Autodesk Fusion 360 part; units mm, degrees
sketch "Sketch1" plane through (0, 0, 0) normal (0, 1, 0) x (1, 0, 0)
  line L0 (-10, 0) -> (17, 0)
  line L1 (17, 0) -> (17, -21.946)
  line L2 (17, -21.946) -> (-10, -21.946)
  line L3 (-10, -21.946) -> (-10, 0)
  dimension "d1" = 21.946
  dimension "d2" = 27
  dimension "d3" = 10
  dimension "d4" = 21.946
extrude "Extrude1" add sketch "Sketch1" along normal blind 5
sketch "Sketch2" plane through (0, 0, 0) normal (0, -1, 0) x (1, 0, 0)
  line L0 (17, 21.946) -> (-10, 21.946)
  line L1 (-10, 21.946) -> (-10, 0)
  line L2 (-10, 0) -> (17, 0)
  line L3 (17, 0) -> (17, 21.946)
  circle A0 centre (3.5, 21.946) radius 13.5
  circle A1 centre (3.5, 21.946) radius 12
  dimension "d7" = 27
  dimension "d8" = 24
extrude "Extrude2" add sketch "Sketch2" against normal blind 5 contours L0 A0 A1 picked at (13.449, 30.2624)
extrude "Extrude3" cut sketch "Sketch2" against normal blind 5 contours L0 A1 picked at (6.689, 16.5654)
equation "d1 = 21.616 mm + 0.33 mm"
equation "d4 = 21.616 mm + 0.33 mm"
Could you check a few things on this model? Use its own coordinates, in mm. Round coordinates to 2 decimals unless told otherwise and drop trailing zeros. Order: outer loops, then holes, each group sorted by start corner. A loop starts at its lowest first (then second) coordinate and runs counter-clockwise, first axis right, second up. Notation, with made-up numbers: M 67,-31.5 L 72,-31.5 A17 ccw 72,-15.5 Z; hole C 29,38.25 d3. An arc over 180 degrees is marked long. One line per item, written item: value.
(1) Imagine slicing it at A-A (x = 3.5). Write out the boundary of the cut face in (y, z), and give its area (3 significant figures).
Ans:
outline: M 0,0 L 5,0 L 5,9.95 L 0,9.95 Z; M 0,33.95 L 5,33.95 L 5,35.45 L 0,35.45 Z
area: 57.2 mm^2
(2) If we mould it in two halves opening along X, with no side actions, what happens to faces 1 (the cylindrical face through (1.938, 2.465, 33.844)), 2 (the flat face through (3.3, 0, 9.6)), 3 (the cylindrical face through (3.797, 2.465, 35.443)), 4 (the flat face through (17, 2, 11))? For each: released by +X, released by -X, zero draft, split by the parting line, or undercut.
Ans:
face 1: undercut
face 2: zero draft
face 3: split by the parting line
face 4: released by +X
(3) I need wall thicknesses on line 1 along Z through (x, y) = (3.5, 2.3); line 2 along Z through (x, y) = (2.75, 3.25); line 3 along X through (y, z) = (4.25, 28.5). Which ranges of each line are inside material? Lowest first, please. Write a range as from..to.
Ans:
line 1: z = 0..9.95, 33.95..35.45
line 2: z = 0..9.97, 33.92..35.43
line 3: x = -8.3..-6.55, 13.55..15.3
(4) Imagine slicing it at C-C (y = 0.65). Write out the boundary of the cut face in (x, z), and give its area (3 significant figures).
Ans:
outline: M -10,0 L 17,0 L 17,21.95 A13.5 ccw -10,21.95 Z; hole C 3.5,21.95 d24
area: 426 mm^2
(5) Imagine slicing it at B-B (z = 14.5). Write out the boundary of the cut face in (x, y).
Ans:
outline: M -10,0 L -5.91,0 L -5.91,5 L -10,5 Z; M 12.91,0 L 17,0 L 17,5 L 12.91,5 Z
